```python
from build123d import *

# Parameters (mm, degrees)
BASE_FLANGE1_DEPTH = 369
CUT_EXTRUDE1_REACH = 376.147
SKETCH2_W          = 20
SKETCH2_H          = 10


# Sheet-metal steps are written as plain solids
with BuildPart() as part:
    # Sketch1 → Base-Flange1 (new, symmetric)
    with BuildSketch(Plane.XY):
        with BuildLine():
            Line((-60, 15), (-31.154700538, 15))
            ThreePointArc((-31.154700538, 15), (-30.154700538, 14.732050808), (-29.422649731, 14))
            Line((-29.422649731, 14), (-22.205771366, 1.5))
            ThreePointArc((-22.205771366, 1.5), (-21.107695155, 0.401923789), (-19.607695155, 0))
            Line((-19.607695155, 0), (19.607695155, 0))
            ThreePointArc((19.607695155, 0), (21.107695155, 0.401923789), (22.205771366, 1.5))
            Line((22.205771366, 1.5), (29.422649731, 14))
            ThreePointArc((29.422649731, 14), (30.154700538, 14.732050808), (31.154700538, 15))
            Line((31.154700538, 15), (60, 15))
            Line((60, 15), (60, 16))
            Line((60, 16), (31.154700538, 16))
            ThreePointArc((31.154700538, 16), (29.654700538, 15.598076211), (28.556624327, 14.5))
            Line((28.556624327, 14.5), (21.339745962, 2))
            ThreePointArc((21.339745962, 2), (20.607695155, 1.267949192), (19.607695155, 1))
            Line((19.607695155, 1), (-19.607695155, 1))
            ThreePointArc((-19.607695155, 1), (-20.607695155, 1.267949192), (-21.339745962, 2))
            Line((-21.339745962, 2), (-28.556624327, 14.5))
            ThreePointArc((-28.556624327, 14.5), (-29.654700538, 15.598076211), (-31.154700538, 16))
            Line((-31.154700538, 16), (-60, 16))
            Line((-60, 16), (-60, 15))
        make_face()
    extrude(amount=BASE_FLANGE1_DEPTH, both=True)

    # Sketch2 → Cut-Extrude1 (cut, up to next)
    with BuildSketch(Plane(origin=(0, 1, 0), x_dir=(1, 0, 0), z_dir=(0, 1, 0)), mode=Mode.PRIVATE) as cut_extrude1_sk1:
        with Locations((0, 364)):
            Rectangle(SKETCH2_W, SKETCH2_H)
    cut_extrude1_tool1 = extrude(cut_extrude1_sk1.sketch, amount=-CUT_EXTRUDE1_REACH, mode=Mode.PRIVATE) & part.part
    # Sketch2 → Cut-Extrude1 (cut, up to next)
    with BuildSketch(Plane(origin=(0, 1, 0), x_dir=(1, 0, 0), z_dir=(0, 1, 0)), mode=Mode.PRIVATE) as cut_extrude1_sk2:
        with Locations((0, -364)):
            Rectangle(SKETCH2_W, SKETCH2_H)
    cut_extrude1_tool2 = extrude(cut_extrude1_sk2.sketch, amount=-CUT_EXTRUDE1_REACH, mode=Mode.PRIVATE) & part.part
    add(cut_extrude1_tool1.solids().sort_by_distance((0, 1, -364))[0], mode=Mode.SUBTRACT)
    add(cut_extrude1_tool2.solids().sort_by_distance((0, 1, 364))[0], mode=Mode.SUBTRACT)


solid = part.part
```
Read the model definition and answer for the solid it produces. Units are mm, in the model's axes. A direction names the side the tool comes from. Give positions to 0.01 mm unless a question says otherwise; leave off trailing zeros. Write each loop counter-clockwise with the first axis right and the second up, starting at its lowest first coordinate (ties: lowest second). Pieces come first, ordered by that corner, then holes. Notation, with made-up numbers: (-18, 60.5) -> (27, 60.5) arc R17 cw to (27, 74.5) -> close; hole circle Ø10 at (0.5, 82). An arc over 180 degrees is marked (long way). Answer in a Markdown table with one row per item.
1) Each of these flat-tipped pins is pushed along its axis until it touches: pin 1 Ø5 at (x, z) = (33.5, -264) entering from -Y; pin 2 Ø1.5 at (x, y) = (-14, 3) entering from -Z; pin 3 Ø1 at (y, z) = (9, 72.5) entering from -X; pin 4 Ø1.1 at (x, y) = (-3.5, 0.5) entering from -Z. Where does it stop, or does it pass through?
Results list:
| item | result |
|---|---|
| pin 1 | y = 14.99 |
| pin 2 | through |
| pin 3 | x = -26.82 |
| pin 4 | z = -359 |
2) Section B-B on z = -180 is taken. Give the vertices of the cut face in (x, y).
Results list:
| item | result |
|---|---|
| outline | (-60, 15) -> (-31.15, 15) arc R2 cw to (-29.42, 14) -> (-22.21, 1.5) arc R3 ccw to (-19.61, 0) -> (19.61, 0) arc R3 ccw to (22.21, 1.5) -> (29.42, 14) arc R2 cw to (31.15, 15) -> (60, 15) -> (60, 16) -> (31.15, 16) arc R3 ccw to (28.56, 14.5) -> (21.34, 2) arc R2 cw to (19.61, 1) -> (-19.61, 1) arc R2 cw to (-21.34, 2) -> (-28.56, 14.5) arc R3 ccw to (-31.15, 16) -> (-60, 16) -> close |
3) Section A-A on y = 8 is taken. Give the vertices of the cut face in (x, z), plus the area to 3 significant figures.
Results list:
| item | result |
|---|---|
| outline | (-25.96, -369) -> (-24.8, -369) -> (-24.8, 369) -> (-25.96, 369) -> close; (24.8, -369) -> (25.96, -369) -> (25.96, 369) -> (24.8, 369) -> close |
| area | 1,700 mm^2 |
4) Determine the mould class of faces 6 (the flat face through (-25.865, 7.837, 5.166)), 7 (the flat face through (25.76, 7.66, 5.17)), 8 (the flat face through (-24.898, 8.163, 5.166)), 9 (the flat face through (46, 16, 5)) for opening direction X: released by +X, released by -X, zero draft, split by the parting line, or undercut.
Results list:
| item | result |
|---|---|
| face 6 | released by -X |
| face 7 | released by +X |
| face 8 | undercut |
| face 9 | zero draft |
5) Straight lines are drawn through the part: line 1 (Y direction, x = 2, z = 224.5); line 2 (Y direction, x = -47, z = -16); line 3 (X direction, y = 12, z = 292). For each, find the intervals that lie inside material, in ascending order. Write a range as [from, to].
Results list:
| item | result |
|---|---|
| line 1 | [0, 1] |
| line 2 | [15, 16] |
| line 3 | [-28.27, -27.11], [27.11, 28.27] |
6) A tool of negligible diameter and unlimited length cuts with its end or side. For faces 1 (the flat face through (34.88, 15.15, -369)), 2 (the flat face through (-45, 16, 5)), 3 (the flat face through (45, 15, 5)), 4 (the flat face through (0, 1, 5)), 5 (the flat face through (-46, 15, 5)), from which of +Z, -Z, +X, -X, +Y, -Y can it reach the whole face along a straight path? Write none if from no direction.
Results list:
| item | result |
|---|---|
| face 1 | -Z, +X, -X, +Y, -Y |
| face 2 | +Z, -Z, +X, -X, +Y |
| face 3 | +Z, -Z, +X, -Y |
| face 4 | +Z, -Z, +Y |
| face 5 | +Z, -Z, -X, -Y |
7) Section C-C on x = -37.5 is taken. Give the vertices of the cut face in (y, z).
Results list:
| item | result |
|---|---|
| outline | (15, -369) -> (16, -369) -> (16, 369) -> (15, 369) -> close |
